Autodesk Inventor part; units mm, degrees
ref_plane "YZ Plane" through (0, 0, 0) normal (1, 0, 0) x (0, 1, 0)
ref_plane "XZ Plane" through (0, 0, 0) normal (0, 1, 0) x (-1, 0, 0)
ref_plane "XY Plane" through (0, 0, 0) normal (0, 0, 1) x (1, 0, 0)
sketch "スケッチ1" plane through (0, 0, 0) normal (0, 0, 1) x (1, 0, 0)
  line L0 (46.5, -40.5) -> (-46.5, -40.5)
  line L1 (-46.5, -40.5) -> (-46.5, 40.5)
  line L2 (-46.5, 40.5) -> (46.5, 40.5)
  line L3 (46.5, 40.5) -> (46.5, -40.5)
  line L4 (46.5, -40.5) -> (-46.5, 40.5) construction
  line L5 (-46.5, -40.5) -> (46.5, 40.5) construction
  point P0 (0, 0)
  dimension "d0" = 93
  dimension "d1" = 81
extrude "押し出し1" add sketch "スケッチ1" along normal blind 1.6
sketch "スケッチ2" plane through (0, 0, 1.6) normal (0, 0, 1) x (1, 0, 0)
  circle A0 centre (-41.5, 35.5) radius 1.6
  line L0 (46.5, 40.5) -> (-46.5, 40.5)
  line L1 (-46.5, 40.5) -> (-46.5, -40.5)
  circle A1 centre (-26.5, -35.5) radius 1.6
  line L2 (-46.5, -40.5) -> (46.5, -40.5)
  circle A2 centre (33.5, -35.5) radius 1.6
  circle A3 centre (0, 20.5) radius 1.6
  point P0 (0, 0)
  dimension "d4" = 3.2
  dimension "d5" = 5
  dimension "d6" = 5
  dimension "d7" = 3.2
  dimension "d8" = 20
  dimension "d9" = 5
  dimension "d11" = 80
  dimension "d14" = 20
extrude "押し出し2" cut sketch "スケッチ2" against normal through all
equation "\"d9\" = d5"
properties part number "board"
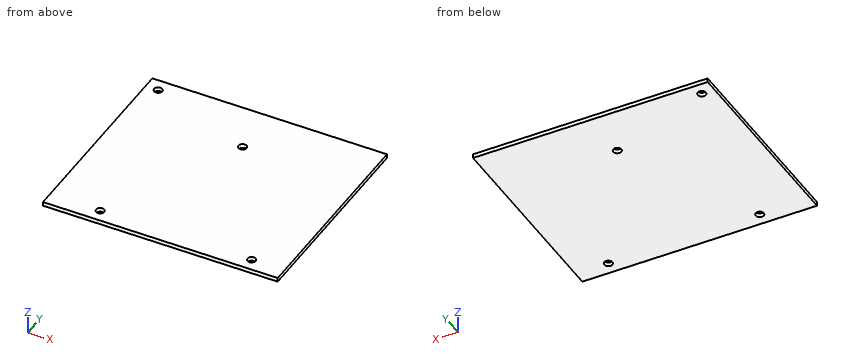
Geometry: final body of the model. Coordinates: model frame, mm. Give positions to 0.01 mm unless a question says otherwise; leave off trailing zeros. Loops run counter-clockwise (first coordinate to the right, second up) from the corner with the lowest first, then second, coordinate; pieces in that order, holes last. Notation, with made-up numbers: M 18,-10 L 63,-10 A22 cw 63,24 Z; hole C 49.25,55.5 d4. An arc over 180 degrees is marked long. Put each result on its own line as item: value.
1) First-contact query: P1, Ø5, axis at x = -41.5, y = 35.5, coming from the +Z side. Flat tip, straight axial feed; report the tip coordinate or a pass-through.
Computed values:
P1: stops at z = 1.6
2) Cut plane C-C, the plane y = -35.5. Return the cut outline in (x, z), plus the area to 3 significant figures.
Computed values:
outline: M -46.5,0 L -28.1,0 L -28.1,1.6 L -46.5,1.6 Z; M -24.9,0 L 31.9,0 L 31.9,1.6 L -24.9,1.6 Z; M 35.1,0 L 46.5,0 L 46.5,1.6 L 35.1,1.6 Z
area: 139 mm^2
3) Material intervals for L1, parallel to Y at x = 33.5, z = 1.25; L2, parallel to Y at x = -41.5, z = 0.6, sorted ascending. Write a range as from..to.
Computed values:
L1: y = -40.5..-37.1, -33.9..40.5
L2: y = -40.5..33.9, 37.1..40.5
4) Cut plane A-A, the plane y = 20.5. Return the cut outline in (x, z), plus the area to 3 significant figures.
Computed values:
outline: M -46.5,0 L -1.6,0 L -1.6,1.6 L -46.5,1.6 Z; M 1.6,0 L 46.5,0 L 46.5,1.6 L 1.6,1.6 Z
area: 144 mm^2
5) Cut plane B-B, the plane x = -41.5. Return the cut outline in (y, z).
Computed values:
outline: M -40.5,0 L 33.9,0 L 33.9,1.6 L -40.5,1.6 Z; M 37.1,0 L 40.5,0 L 40.5,1.6 L 37.1,1.6 Z
